Autodesk Inventor part; units mm, degrees
ref_plane "YZ Plane" through (0, 0, 0) normal (1, 0, 0) x (0, 1, 0)
ref_plane "XZ Plane" through (0, 0, 0) normal (0, 1, 0) x (-1, 0, 0)
ref_plane "XY Plane" through (0, 0, 0) normal (0, 0, 1) x (1, 0, 0)
sketch "Sketch1" plane through (0, 0, 0) normal (0, 1, 0) x (-1, 0, 0)
  line L0 (4, 59.5) -> (-4, 59.5)
  line L1 (-4, 59.5) -> (-4, -59.5)
  line L2 (-4, -59.5) -> (4, -59.5)
  line L3 (4, -59.5) -> (4, 59.5)
  line L4 (4, 59.5) -> (-4, -59.5) construction
  line L5 (-4, 59.5) -> (4, -59.5) construction
  point P0 (0, 0)
  dimension "d0" = 8
  dimension "d1" = 119
extrude "Extrusion1" add sketch "Sketch1" along normal blind 8
sketch "Sketch2" plane through (0, 8, 0) normal (0, 1, 0) x (1, 0, 0)
  line L0 (-9, -41) -> (1, -41)
  line L1 (1, -41) -> (1, 41)
  line L2 (1, 41) -> (-9, 41)
  line L3 (-9, 41) -> (-9, -41)
  line L4 (-4, 59.5) -> (-4, -59.5)
  line L5 (-9, -41) -> (1, 41) construction
  line L6 (1, -41) -> (-9, 41) construction
  point P0 (0, 0)
  point P1 (-4, 0)
  dimension "d4" = 10
  dimension "d5" = 82
extrude "Extrusion2" cut sketch "Sketch2" against normal blind 8
sketch "Sketch3" plane through (-4, 0, 59.5) normal (0, 0, 1) x (1, 0, 0)
  circle A0 centre (4, 4) radius 1.5
  line L0 (0, 8) -> (8, 8)
  line L1 (8, 0) -> (8, 8)
  dimension "d8" = 3
  dimension "d31" = 4
  dimension "d32" = 4
hole "Hole1" at (0, 4, 59.5) direction (0, 0, -1) diameter 3 depth 8 tip angle 118
thread "Thread1"
sketch "Sketch4" plane through (4, 0, -59.5) normal (0, 0, -1) x (-1, 0, 0)
  circle A0 centre (4, 4) radius 1.5
  line L0 (0, 8) -> (8, 8)
  line L1 (0, 0) -> (0, 8)
  dimension "d19" = 3
  dimension "d33" = 4
  dimension "d34" = 4
hole "Hole2" at (0, 4, -59.5) direction (0, 0, 1) diameter 3 depth 8 tip angle 118
thread "Thread2"
properties part number "TopSupportPlate"
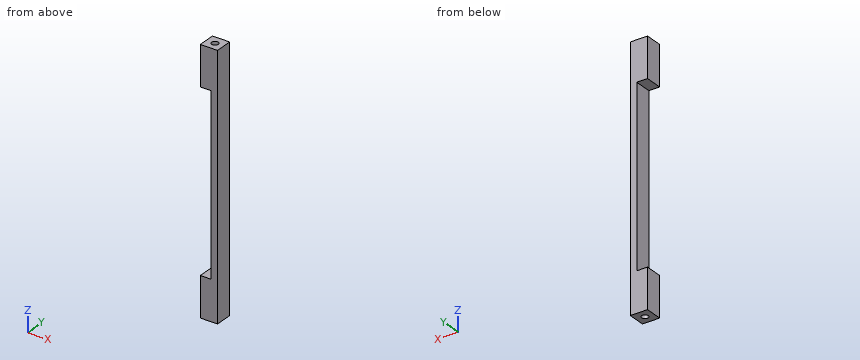
Part model, mm, in its own coordinate system. Coordinates: 2 decimals unless noted, no trailing zeros. Order: outer loops, then holes, each group sorted by start corner. A loop starts at its lowest first (then second) coordinate and runs counter-clockwise, first axis right, second up.
(1) Slice it at A-A, the plane x = -3. Write the cut outline in (y, z).
Check sheet entries:
outline: (0, -59.5) - (8, -59.5) - (8, -41) - (0, -41) - close; (0, 41) - (8, 41) - (8, 59.5) - (0, 59.5) - close
(2) Pin check, flat tips, straight feed: pin 1 Ø3.5 at (x, y) = (0, 4) entering from -Z; pin 2 Ø3 at (x, z) = (-1, -26) entering from -Y; pin 3 Ø1.8 at (x, y) = (0, 4) entering from -Z. Stop position of each tip, or through.
Check sheet entries:
pin 1: stops at z = -59.5
pin 2: passes through
pin 3: stops at z = -51.14
(3) Probe L1, parallel to Y at x = 0, z = -54.75; L2, parallel to Z at x = -2.75, y = 3; L3, parallel to X at y = 3.75, z = 52. List the from-to ranges inside material, lowest first.
Check sheet entries:
L1: y = 0 to 2.5, 5.5 to 8
L2: z = -59.5 to -41, 41 to 59.5
L3: x = -4 to -1.48, 1.48 to 4
(4) Slice it at B-B, the plane z = -12. Write the cut outline in (x, y), and give its area (3 significant figures).
Check sheet entries:
outline: (1, 0) - (4, 0) - (4, 8) - (1, 8) - close
area: 24.0 mm2
